Here's how the part is built. I have some questions about the finished solid (model axes, mm). Face numbers are marked on the shaded views. A direction names the side the tool comes from. Coordinates: 2 decimals unless noted, no trailing zeros. Write each loop counter-clockwise with the first axis right and the second up, starting at its lowest first coordinate (ties: lowest second). Pieces come first, ordered by that corner, then holes.
(1) Imagine slicing it at A-A, the plane x = 45.5. List the corners of the cut face in (y, z) for me, plus the area to 3 significant figures.
(2) Imagine slicing it at B-B, the plane z = 33. List the corners of the cut face in (x, y) for me, plus the area to 3 significant figures.
(3) For pin 1 Ø5.5 at (x, y) = (20.5, -25) entering from +Z; pin 2 Ø4 at (x, y) = (-6.5, 3) entering from -Z; pin 3 Ø8 at (y, z) = (23.5, 20) entering from +X, each with a flat end and sliding along its axis, tell me the tip position at first contact or that it passes through.
(4) Imagine slicing it at D-D, the plane z = 65. List the corners of the cut face in (x, y) for me, plus the area to 3 significant figures.
(5) Imagine slicing it at C-C, the plane y = 14. List the corners of the cut face in (x, z) for me, plus the area to 3 significant figures.
(6) Please list where these lines run through material, in increasing order: probe 1 along Y at (x, z) = (62.4, -4); probe 2 along X at (y, z) = (-3, 20); probe 3 along Y at (x, z) = (22, -3.5).
(7) Which directions (+Z, -Z, +X, -X, +Y, -Y) give clear straight access to the entire face, cutting with the end or side of a thin tool? Please do the marked faces 1, 2, 3, 4 and 5.
(8) Thinking about a two-plate mould opening in Y: for the marked faces 6, 7 and 8, which applies, released by +Y, released by -Y, zero draft, split by the parting line, or undercut?
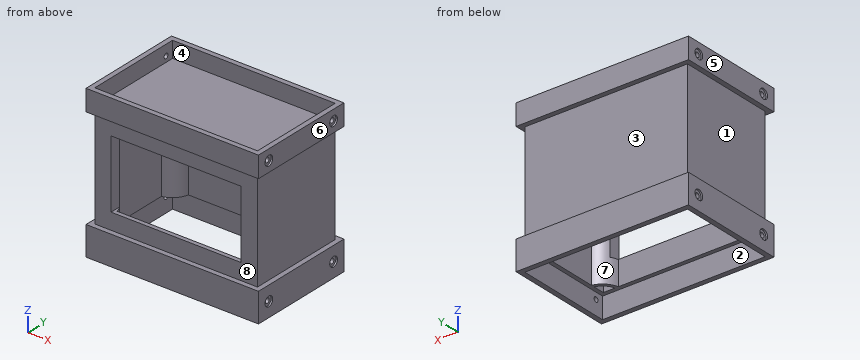
```python
from build123d import *

# Parameters (mm, degrees)
SKETCH1_W                = 100
SKETCH1_H                = 60
SKETCH1_W_2              = 95
SKETCH1_H_2              = 55
BOSS_EXTRUDE1_DEPTH      = 150
SKETCH2_W                = 95
SKETCH2_H                = 15
CUT_EXTRUDE1_DEPTH       = 20
BOSS_EXTRUDE2_DEPTH      = 13
BOSS_EXTRUDE2_DEPTH_BACK = 5
SKETCH3_W                = 106
SKETCH3_H                = 66
SKETCH3_W_2              = 100
SKETCH3_H_2              = 60
SKETCH4_R                = 1.5
CUT_EXTRUDE2_DEPTH       = 120
SKETCH5_R                = 3
CUT_EXTRUDE3_DEPTH       = 1
CUT_EXTRUDE4_START       = -1
SKETCH6_R                = 3
CUT_EXTRUDE4_DEPTH       = 1
SKETCH8_W                = 125.879436885
SKETCH8_H                = 80.445742456
CUT_EXTRUDE6_DEPTH       = 80
BOSS_EXTRUDE3_DEPTH      = 10
BOSS_EXTRUDE3_DEPTH_BACK = 3
SKETCH9_W                = 106
SKETCH9_H                = 66
SKETCH9_W_2              = 100
SKETCH9_H_2              = 60
SKETCH10_R               = 1.5
CUT_EXTRUDE7_DEPTH       = 117
SKETCH10_3_R             = 3
CUT_EXTRUDE8_DEPTH       = 1
CUT_EXTRUDE9_START       = -1
SKETCH11_R               = 3
CUT_EXTRUDE9_DEPTH       = 1
SKETCH12_W               = 100
SKETCH12_H               = 60
BOSS_EXTRUDE4_DEPTH      = 2
SKETCH13_W               = 80
SKETCH13_H               = 42
CUT_EXTRUDE10_DEPTH      = 10


with BuildPart() as part:
    # Sketch1 → Boss-Extrude1 (new body)
    # profile 1 of 5: a face of its own
    with BuildSketch(Plane.XY):
        with Locations((9.751655629, 0.960264901)):
            Rectangle(SKETCH1_W, SKETCH1_H)
        with Locations((9.751655629, 0.960264901)):
            Rectangle(SKETCH1_W_2, SKETCH1_H_2, mode=Mode.SUBTRACT)
    # profile 2 of 5: a face of its own
    with BuildSketch(Plane.XY):
        with BuildLine():
            Line((-28.511649777, 28.460264901), (-30.565886005, 28.460264901))
            ThreePointArc((-30.565886005, 28.460264901), (-33.177276559, 23.889197089), (-37.748344371, 21.277806535))
            Line((-37.748344371, 21.277806535), (-37.748344371, 19.223570306))
            ThreePointArc((-37.748344371, 19.223570306), (-31.763062997, 22.474983526), (-28.511649777, 28.460264901))
        make_face()
    # profile 3 of 5: a face of its own
    with BuildSketch(Plane.XY):
        with BuildLine():
            Line((50.069197264, 28.460264901), (48.014961035, 28.460264901))
            ThreePointArc((48.014961035, 28.460264901), (51.266374255, 22.474983526), (57.251655629, 19.223570306))
            Line((57.251655629, 19.223570306), (57.251655629, 21.277806535))
            ThreePointArc((57.251655629, 21.277806535), (52.680587817, 23.889197089), (50.069197264, 28.460264901))
        make_face()
    # profile 4 of 5: a face of its own
    with BuildSketch(Plane.XY):
        with BuildLine():
            Line((57.251655629, -19.357276734), (57.251655629, -17.303040505))
            ThreePointArc((57.251655629, -17.303040505), (51.266374255, -20.554453725), (48.014961035, -26.539735099))
            Line((48.014961035, -26.539735099), (50.069197264, -26.539735099))
            ThreePointArc((50.069197264, -26.539735099), (52.680587817, -21.968667287), (57.251655629, -19.357276734))
        make_face()
    # profile 5 of 5: a face of its own
    with BuildSketch(Plane.XY):
        with BuildLine():
            ThreePointArc((-28.511649777, -26.539735099), (-31.763062997, -20.554453725), (-37.748344371, -17.303040505))
            Line((-37.748344371, -17.303040505), (-37.748344371, -19.357276734))
            ThreePointArc((-37.748344371, -19.357276734), (-33.177276559, -21.968667287), (-30.565886005, -26.539735099))
            Line((-30.565886005, -26.539735099), (-28.511649777, -26.539735099))
        make_face()
    extrude(amount=BOSS_EXTRUDE1_DEPTH)

    # Sketch2 → Cut-Extrude1 (cut)
    with BuildSketch(Plane(origin=(0, 30.960264901, 0), x_dir=(1, 0, 0), z_dir=(0, 1, 0))):
        with Locations((9.751655629, -142.5)):
            Rectangle(SKETCH2_W, SKETCH2_H)
    extrude(amount=-CUT_EXTRUDE1_DEPTH, mode=Mode.SUBTRACT)

    # Sketch3 → Boss-Extrude2 (add, two sides: drawn at the far end of the back side and taken through both)
    with BuildSketch(Plane(origin=(0, 0, 0), x_dir=(-1, 0, 0), z_dir=(0, 0, -1)).offset(-BOSS_EXTRUDE2_DEPTH_BACK)):
        with Locations((-9.751655629, 0.960264901)):
            Rectangle(SKETCH3_W, SKETCH3_H)
        with Locations((-9.751655629, 0.960264901)):
            Rectangle(SKETCH3_W_2, SKETCH3_H_2, mode=Mode.SUBTRACT)
    extrude(amount=BOSS_EXTRUDE2_DEPTH + BOSS_EXTRUDE2_DEPTH_BACK)

    # Sketch4 → Cut-Extrude2 (cut)
    with BuildSketch(Plane.ZY.offset(43.248344371)):
        with Locations((-4, -24.039735099)):
            Circle(SKETCH4_R)
        with Locations((-4, 25.960264901)):
            Circle(SKETCH4_R)
    extrude(amount=-CUT_EXTRUDE2_DEPTH, mode=Mode.SUBTRACT)

    # Sketch5 → Cut-Extrude3 (cut)
    with BuildSketch(Plane(origin=(62.751655629, 0, 0), x_dir=(0, 0, -1), z_dir=(1, 0, 0))):
        with Locations((4, -24.039735099)):
            Circle(SKETCH5_R)
        with Locations((4, 25.960264901)):
            Circle(SKETCH5_R)
    extrude(amount=-CUT_EXTRUDE3_DEPTH, mode=Mode.SUBTRACT)

    # Sketch6 → Cut-Extrude4 (cut)
    with BuildSketch(Plane.ZY.offset(43.248344371).offset(CUT_EXTRUDE4_START)):
        with Locations(Location((-4, 25.960264901, 0), (0, 0, 180))):
            Circle(SKETCH6_R)
        with Locations((-4, -24.087684502)):
            Circle(SKETCH6_R)
    extrude(amount=CUT_EXTRUDE4_DEPTH, mode=Mode.SUBTRACT)

    # Sketch8 → Cut-Extrude6 (cut)
    with BuildSketch(Plane.XY.offset(150)):
        with Locations((7.819552644, 0.433327723)):
            Rectangle(SKETCH8_W, SKETCH8_H)
    extrude(amount=-CUT_EXTRUDE6_DEPTH, mode=Mode.SUBTRACT)

    # Sketch9 → Boss-Extrude3 (add, two sides: drawn at the far end of the back side and taken through both)
    with BuildSketch(Plane.XY.offset(70).offset(-BOSS_EXTRUDE3_DEPTH_BACK)):
        with Locations((9.751655629, 0.960264901)):
            Rectangle(SKETCH9_W, SKETCH9_H)
        with Locations((9.751655629, 0.960264901)):
            Rectangle(SKETCH9_W_2, SKETCH9_H_2, mode=Mode.SUBTRACT)
    extrude(amount=BOSS_EXTRUDE3_DEPTH + BOSS_EXTRUDE3_DEPTH_BACK)

    # Sketch10 → Cut-Extrude7 (cut)
    with BuildSketch(Plane.ZY.offset(43.248344371)):
        with Locations(Location((73.5, 25.960264901, 0), (0, 0, 180))):
            Circle(SKETCH10_R)
        with Locations(Location((73.5, -24.039735099, 0), (0, 0, 180))):
            Circle(SKETCH10_R)
    extrude(amount=-CUT_EXTRUDE7_DEPTH, mode=Mode.SUBTRACT)

    # Sketch10_3 → Cut-Extrude8 (cut)
    with BuildSketch(Plane.ZY.offset(43.248344371)):
        with Locations((73.5, 25.960264901)):
            Circle(SKETCH10_3_R)
        with Locations((73.5, -24.039735099)):
            Circle(SKETCH10_3_R)
    extrude(amount=-CUT_EXTRUDE8_DEPTH, mode=Mode.SUBTRACT)

    # Sketch11 → Cut-Extrude9 (cut)
    with BuildSketch(Plane(origin=(62.751655629, 0, 0), x_dir=(0, 0, -1), z_dir=(1, 0, 0)).offset(CUT_EXTRUDE9_START)):
        with Locations(Location((-73.5, -24.039735099, 0), (0, 0, 180))):
            Circle(SKETCH11_R)
        with Locations(Location((-73.5, 25.960264901, 0), (0, 0, 180))):
            Circle(SKETCH11_R)
    extrude(amount=CUT_EXTRUDE9_DEPTH, mode=Mode.SUBTRACT)

    # Sketch12 → Boss-Extrude4 (add)
    with BuildSketch(Plane.XY.offset(70)):
        with Locations((9.751655629, 0.960264901)):
            Rectangle(SKETCH12_W, SKETCH12_H)
    extrude(amount=-BOSS_EXTRUDE4_DEPTH)

    # Sketch13 → Cut-Extrude10 (cut)
    with BuildSketch(Plane.XZ.offset(29.039735099)):
        with Locations((9.751655629, 36)):
            Rectangle(SKETCH13_W, SKETCH13_H)
    extrude(amount=-CUT_EXTRUDE10_DEPTH, mode=Mode.SUBTRACT)


solid = part.part
```
Recorded:
1. outline: (-32.04, -13) - (-29.04, -13) - (-29.04, 0) - (-26.54, 0) - (-26.54, 15) - (-29.04, 15) - (-29.04, 5) - (-32.04, 5) - close; (-32.04, 67) - (-29.04, 67) - (-29.04, 57) - (-26.54, 57) - (-26.54, 68) - (28.46, 68) - (28.46, 0) - (30.96, 0) - (30.96, -13) - (33.96, -13) - (33.96, 5) - (30.96, 5) - (30.96, 67) - (33.96, 67) - (33.96, 80) - (30.96, 80) - (30.96, 70) - (-29.04, 70) - (-29.04, 80) - (-32.04, 80) - close
1. area: 541 mm2
2. outline: (-40.25, -29.04) - (-30.25, -29.04) - (-30.25, -22.41) arc R12 ccw to (-37.75, -17.3) - (-37.75, 19.22) arc R12 ccw to (-28.51, 28.46) - (48.01, 28.46) arc R12 ccw to (57.25, 19.22) - (57.25, -17.3) arc R12 ccw to (49.75, -22.41) - (49.75, -29.04) - (59.75, -29.04) - (59.75, 30.96) - (-40.25, 30.96) - close; hole (-37.75, -26.54) - (-30.57, -26.54) arc R10 ccw to (-37.75, -19.36) - close; hole (-37.75, 21.28) arc R10 ccw to (-30.57, 28.46) - (-37.75, 28.46) - close; hole (50.07, -26.54) - (57.25, -26.54) - (57.25, -19.36) arc R10 ccw to start; hole (50.07, 28.46) arc R10 ccw to (57.25, 21.28) - (57.25, 28.46) - close
2. area: 664 mm2
3. pin 1: stops at z = 70
3. pin 2: stops at z = 68
3. pin 3: stops at x = 59.75
4. outline: (-40.25, -29.04) - (59.75, -29.04) - (59.75, 30.96) - (-40.25, 30.96) - close; hole (-37.75, -26.54) - (-30.57, -26.54) arc R10 ccw to (-37.75, -19.36) - close; hole (-37.75, -17.3) arc R12 cw to (-28.51, -26.54) - (48.01, -26.54) arc R12 cw to (57.25, -17.3) - (57.25, 19.22) arc R12 cw to (48.01, 28.46) - (-28.51, 28.46) arc R12 cw to (-37.75, 19.22) - close; hole (-37.75, 21.28) arc R10 ccw to (-30.57, 28.46) - (-37.75, 28.46) - close; hole (50.07, -26.54) - (57.25, -26.54) - (57.25, -19.36) arc R10 ccw to start; hole (50.07, 28.46) arc R10 ccw to (57.25, 21.28) - (57.25, 28.46) - close
4. area: 873 mm2
5. outline: (-43.25, -13) - (-40.25, -13) - (-40.25, 0) - (-37.75, 0) - (-37.75, 68) - (57.25, 68) - (57.25, 0) - (59.75, 0) - (59.75, -13) - (62.75, -13) - (62.75, 5) - (59.75, 5) - (59.75, 67) - (62.75, 67) - (62.75, 80) - (59.75, 80) - (59.75, 70) - (-40.25, 70) - (-40.25, 80) - (-43.25, 80) - (-43.25, 67) - (-40.25, 67) - (-40.25, 5) - (-43.25, 5) - close
5. area: 726 mm2
6. probe 1: y = -32.04 to -27.04, -21.04 to 22.96, 28.96 to 33.96
6. probe 2: x = -40.25 to -37.75, 57.25 to 59.75
6. probe 3: y = -32.04 to -29.04, 30.96 to 33.96
7. face 1: -X, +Y, -Y
7. face 2: -Z
7. face 3: +X, -X, +Y
7. face 4: +Z
7. face 5: +Z, -Z, -X, +Y, -Y
8. face 6: zero draft
8. face 7: undercut
8. face 8: released by -Y
